Geometry check sheet. Reference: the model listing, model coordinates, mm. A direction names the side the tool comes from. Coordinates: 2 decimals unless noted, no trailing zeros. Loops run counter-clockwise (first coordinate to the right, second up) from the corner with the lowest first, then second, coordinate; pieces in that order, holes last.
from build123d import *

# Parameters (mm, degrees)
SKETCH1_W                    = 400
SKETCH1_H                    = 100
BASE_DEPTH                   = 12
PART_TAPE_MOVER_CUTOUT_DEPTH = 13
PRESS_PLATE_CUTOUT_DEPTH     = 13
ROLLER_CUTOUT_DEPTH          = 13
SKETCH5_W                    = 315.5
SKETCH5_H                    = 8
PART_TAPE_CUTOUT_DEPTH       = 5.5
SKETCH6_W                    = 315.5
SKETCH6_H                    = 12
CUT_EXTRUDE5_DEPTH           = 1
SKETCH9_R                    = 2.065
CUT_EXTRUDE8_DEPTH           = 10
CUT_EXTRUDE9_DEPTH           = 5
CUT_EXTRUDE10_DEPTH          = 8
LPATTERN1_COUNT              = 2
LPATTERN1_PITCH              = 84
LPATTERN1_COUNT_DIR2         = 2
LPATTERN1_PITCH_DIR2         = 40
SKETCH13_R                   = 3
CUT_EXTRUDE11_DEPTH          = 3.5
SKETCH14_R                   = 1.5
CUT_EXTRUDE12_DEPTH          = 9.5
LPATTERN2_COUNT              = 2
LPATTERN2_PITCH              = 48
SKETCH15_R                   = 1.23
CUT_EXTRUDE13_DEPTH          = 13
SKETCH16_R                   = 2.065
CUT_EXTRUDE14_DEPTH          = 13
SKETCH18_R                   = 1.62
CUT_EXTRUDE15_DEPTH          = 13
SKETCH19_R                   = 2.065
SKETCH19_R_2                 = 1.62
CUT_EXTRUDE16_DEPTH          = 8


with BuildPart() as part:
    # Sketch1 → Base (new body)
    with BuildSketch(Plane.XY):
        Rectangle(SKETCH1_W, SKETCH1_H)
    extrude(amount=BASE_DEPTH)

    # Sketch2 → Part Tape Mover Cutout (cut, through all)
    with BuildSketch(Plane.XY.offset(12)):
        with BuildLine():
            Line((200, 0), (149, 0))
            ThreePointArc((149, 0), (146.525126266, 1.025126266), (145.5, 3.5))
            Line((145.5, 3.5), (145.5, 36.5))
            ThreePointArc((145.5, 36.5), (146.525126266, 38.974873734), (149, 40))
            Line((149, 40), (200, 40))
            Line((200, 40), (200, 0))
        make_face()
    extrude(amount=-PART_TAPE_MOVER_CUTOUT_DEPTH, mode=Mode.SUBTRACT)

    # Sketch3 → Press Plate Cutout (cut, through all)
    with BuildSketch(Plane.XY.offset(12)):
        with BuildLine():
            Line((41.5, -10), (103.5, -10))
            ThreePointArc((103.5, -10), (105.974873734, -8.974873734), (107, -6.5))
            Line((107, -6.5), (107, 50))
            Line((107, 50), (38, 50))
            Line((38, 50), (38, -6.5))
            ThreePointArc((38, -6.5), (39.025126266, -8.974873734), (41.5, -10))
        make_face()
    extrude(amount=-PRESS_PLATE_CUTOUT_DEPTH, mode=Mode.SUBTRACT)

    # Sketch4 → Roller Cutout (cut, through all)
    with BuildSketch(Plane.XY.offset(12)):
        with BuildLine():
            Line((-200, 40), (-173.5, 40))
            ThreePointArc((-173.5, 40), (-171.025126266, 38.974873734), (-170, 36.5))
            Line((-170, 36.5), (-170, 3.5))
            ThreePointArc((-170, 3.5), (-171.025126266, 1.025126266), (-173.5, 0))
            Line((-173.5, 0), (-200, 0))
            Line((-200, 0), (-200, 40))
        make_face()
    extrude(amount=-ROLLER_CUTOUT_DEPTH, mode=Mode.SUBTRACT)

    # Sketch5 → Part Tape Cutout (cut)
    with BuildSketch(Plane.XY.offset(12)):
        with Locations((-12.25, 19)):
            Rectangle(SKETCH5_W, SKETCH5_H)
    extrude(amount=-PART_TAPE_CUTOUT_DEPTH, mode=Mode.SUBTRACT)

    # Sketch6 → Cut-Extrude5 (cut)
    with BuildSketch(Plane.XY.offset(12)):
        with Locations((-12.25, 18)):
            Rectangle(SKETCH6_W, SKETCH6_H)
    extrude(amount=-CUT_EXTRUDE5_DEPTH, mode=Mode.SUBTRACT)

    # Sketch9 → Cut-Extrude8 (cut)
    with BuildSketch(Plane(origin=(0, 50, 0), x_dir=(1, 0, 0), z_dir=(0, 1, 0))):
        with Locations((141, -6)):
            Circle(SKETCH9_R)
        with Locations((192, -6)):
            Circle(SKETCH9_R)
    extrude(amount=-CUT_EXTRUDE8_DEPTH, mode=Mode.SUBTRACT)

    # Sketch11 → Cut-Extrude9 (cut)
    with BuildSketch(Plane.XY.offset(12)):
        with BuildLine():
            Line((110.25, 35), (110.25, 45))
            ThreePointArc((110.25, 45), (114.5, 49.25), (118.75, 45))
            Line((118.75, 45), (118.75, 35))
            ThreePointArc((118.75, 35), (114.5, 30.75), (110.25, 35))
        make_face()
    cut_extrude9 = extrude(amount=-CUT_EXTRUDE9_DEPTH, mode=Mode.SUBTRACT)

    # Sketch12 → Cut-Extrude10 (cut, through all)
    with BuildSketch(Plane.XY.offset(7)):
        with BuildLine():
            Line((117.25, 35), (117.25, 45))
            ThreePointArc((117.25, 45), (114.5, 47.75), (111.75, 45))
            Line((111.75, 45), (111.75, 35))
            ThreePointArc((111.75, 35), (114.5, 32.25), (117.25, 35))
        make_face()
    cut_extrude10 = extrude(amount=-CUT_EXTRUDE10_DEPTH, mode=Mode.SUBTRACT)

    # LPattern1: Cut-Extrude9, Cut-Extrude10 2 × 2
    with Locations(*[(-i * LPATTERN1_PITCH, -j * LPATTERN1_PITCH_DIR2, 0) for i in range(LPATTERN1_COUNT) for j in range(LPATTERN1_COUNT_DIR2) if (i, j) != (0, 0)]):
        add(cut_extrude9, mode=Mode.SUBTRACT)
        add(cut_extrude10, mode=Mode.SUBTRACT)

    # Sketch13 → Cut-Extrude11 (cut)
    with BuildSketch(Plane.XY.offset(12)):
        with Locations((-181, 44)):
            Circle(SKETCH13_R)
        with Locations((-195, 44)):
            Circle(SKETCH13_R)
    cut_extrude11 = extrude(amount=-CUT_EXTRUDE11_DEPTH, mode=Mode.SUBTRACT)

    # Sketch14 → Cut-Extrude12 (cut, through all)
    with BuildSketch(Plane.XY.offset(8.5)):
        with Locations((-181, 44)):
            Circle(SKETCH14_R)
        with Locations((-195, 44)):
            Circle(SKETCH14_R)
    cut_extrude12 = extrude(amount=-CUT_EXTRUDE12_DEPTH, mode=Mode.SUBTRACT)

    # LPattern2: Cut-Extrude11, Cut-Extrude12 ×2
    with Locations(*[(0, -i * LPATTERN2_PITCH, 0) for i in range(1, LPATTERN2_COUNT)]):
        add(cut_extrude11, mode=Mode.SUBTRACT)
        add(cut_extrude12, mode=Mode.SUBTRACT)

    # Sketch15 → Cut-Extrude13 (cut, through all)
    with BuildSketch(Plane.XY.offset(12)):
        with Locations((-164.15, 40.25)):
            Circle(SKETCH15_R)
        with Locations((-164.15, 0.25)):
            Circle(SKETCH15_R)
        with Locations((-117.5, 4.3)):
            Circle(SKETCH15_R)
    extrude(amount=-CUT_EXTRUDE13_DEPTH, mode=Mode.SUBTRACT)

    # Sketch16 → Cut-Extrude14 (cut, through all)
    with BuildSketch(Plane.XY.offset(12)):
        with Locations((-140, 30.25)):
            Circle(SKETCH16_R)
        with Locations((-100, 30.25)):
            Circle(SKETCH16_R)
    extrude(amount=-CUT_EXTRUDE14_DEPTH, mode=Mode.SUBTRACT)

    # Sketch18 → Cut-Extrude15 (cut, through all)
    with BuildSketch(Plane.XY.offset(12)):
        with Locations((8, 32.5)):
            Circle(SKETCH18_R)
        with Locations((8, 4)):
            Circle(SKETCH18_R)
    extrude(amount=-CUT_EXTRUDE15_DEPTH, mode=Mode.SUBTRACT)

    # Sketch19 → Cut-Extrude16 (cut)
    with BuildSketch(Plane(origin=(0, 50, 0), x_dir=(1, 0, 0), z_dir=(0, 1, 0))):
        with Locations((24, -6)):
            Circle(SKETCH19_R)
        with Locations((4, -6)):
            Circle(SKETCH19_R)
        with Locations((-110, -6)):
            Circle(SKETCH19_R_2)
        with Locations((-150, -6)):
            Circle(SKETCH19_R_2)
    extrude(amount=-CUT_EXTRUDE16_DEPTH, mode=Mode.SUBTRACT)


solid = part.part
1) Section check B-B on x = 13.5. Record the cut outline in (y, z), and give its area (3 significant figures).
Data:
outline: (-50, 0) - (50, 0) - (50, 12) - (24, 12) - (24, 11) - (23, 11) - (23, 6.5) - (15, 6.5) - (15, 11) - (12, 11) - (12, 12) - (-50, 12) - close
area: 1,150 mm2
2) Section check A-A on x = 172.5. Record the cut outline in (y, z), and give its area (3 significant figures).
Data:
outline: (-50, 0) - (0, 0) - (0, 12) - (-50, 12) - close; (40, 0) - (50, 0) - (50, 12) - (40, 12) - close
area: 720 mm2
3) Material ranges on probe 1 along X at (y, z) = (35.5, 6.25); probe 2 along Y at (x, z) = (-181, 9.3); probe 3 along Y at (x, z) = (-109.5, 7.75), recorded low to high.
Data:
probe 1: x = -170 to 27.75, 33.25 to 38, 107 to 111.75, 117.25 to 145.5
probe 2: y = -50 to -7, -1 to 0, 40 to 41, 47 to 50
probe 3: y = -50 to 15, 23 to 50
4) Depth check by flat-ended pin: pin 1 (1 mm diameter, centred on y = 24.5, z = 10.5, fed in from +X); pin 2 (1 mm diameter, centred on x = -110.5, z = 6, fed in from +Y); pin 3 (2 mm diameter, centred on y = 18.5, z = 9, fed in from +X); pin 4 (4 mm diameter, centred on x = -195, y = 44, fed in from +Z). Enter the tip coordinate at first touch or a pass-through.
Data:
pin 1: stops at x = 145.5
pin 2: stops at y = 42
pin 3: passes through
pin 4: stops at z = 8.5
5) Mould release check, pull along X, two halves, no side actions. Record for faces 4 (the flat face through (117.25, 40, 4)), 5 (the flat face through (-3, -10, 0)), 6 (the flat face through (200, 45, 6)): +X half, -X half, draft (parallel to the pull), parting line (faces both ways), or undercut.
Data:
face 4: undercut
face 5: draft
face 6: +X half
6) Access from +Z, -Z, +X, -X, +Y, -Y to the whole of each face (thin tool, end or side, straight path). Record for faces 1 (the flat face through (33.25, 40, 4)), 2 (the flat face through (117.4, 0.1, 7)), 3 (the flat face through (145.5, 20, 6)).
Data:
face 1: +Z, -Z
face 2: +Z
face 3: +Z, -Z, +X
